Geometry check sheet. Reference: the model listing, model coordinates, mm. Give positions to 0.01 mm unless a question says otherwise; leave off trailing zeros. Order: outer loops, then holes, each group sorted by start corner. A loop starts at its lowest first (then second) coordinate and runs counter-clockwise, first axis right, second up. Notation, with made-up numbers: (-21, 79) - (20, 79) arc R28 ccw to (20, 116) - close; hole circle Ø4 at (-9.75, 61.25). An arc over 180 degrees is marked (long way). Put each result on its own line as item: value. Start each with the question number.
```python
from build123d import *

# Parameters (mm, degrees)
F0_W     = 285.75
F0_H     = 50.8
F0_R     = 2.5527
F1_DEPTH = 3.175
F3_DEPTH = 285.751


with BuildPart() as f1:
    # F0 (on Top) → F1 (new body)
    with BuildSketch(Plane.XY):
        with Locations((142.875, -25.4)):
            Rectangle(F0_W, F0_H)
        with Locations((25.4, -38.1)):
            Circle(F0_R, mode=Mode.SUBTRACT)
        with Locations((260.35, -38.1)):
            Circle(F0_R, mode=Mode.SUBTRACT)
        with Locations((25.4, -12.7)):
            Circle(F0_R, mode=Mode.SUBTRACT)
        with Locations((260.35, -12.7)):
            Circle(F0_R, mode=Mode.SUBTRACT)
    extrude(amount=F1_DEPTH)

    # F2 (on face) → F3 (cut, through all)
    with BuildSketch(Plane.YZ.offset(285.75)):
        Polygon((-50.8, 3.175), (-50.8, 0), (-34.366313, 3.175), align=None)
    extrude(amount=-F3_DEPTH, mode=Mode.SUBTRACT)


solid = f1.part
```
Item 1: Cross-section at C-C (y = -38.1). Enter the section's corners in (x, z).
Item 2: Cross-section at B-B (z = 1). Enter the section's corners in (x, y), and give its area (3 significant figures).
Item 3: Thickness scan on line 1 along X through (y, z) = (-38.1, 1.35); line 2 along X through (y, z) = (-12.5, 0.25); line 3 along Y through (x, z) = (25.4, 2.3). Record the ranges inside material, lowest first.
Item 4: Release check for a two-part mould opening along X. For faces 1 (the face through (25.07, -35.57, 1.16)), 2 (the face through (144.875, -42.698, 1.565)) record: +X half, -X half, draft (parallel to the pull), parting line (faces both ways), or undercut.
Item 5: Cross-section at A-A (x = 260.35). Enter the section's corners in (y, z) (3 decimals), and give its area (3 significant figures).
Item 6: Cross-section at D-D (x = 54.5). Enter the section's corners in (y, z) (3 decimals), and give its area (3 significant figures).
Item 7: Gauge pin test, flat end, axial feed: pin 1 Ø4.5 at (x, y) = (25.4, -38.1) entering from -Z. Record the tip position at first contact, or that the pin passes through.
Recorded:
1. outline: (0, 0) - (22.85, 0) - (22.85, 2.45) - (0, 2.45) - close; (27.95, 0) - (257.8, 0) - (257.8, 2.45) - (27.95, 2.45) - close; (262.9, 0) - (285.75, 0) - (285.75, 2.45) - (262.9, 2.45) - close
2. outline: (0, -45.62) - (285.75, -45.62) - (285.75, 0) - (0, 0) - close; hole circle Ø5.11 at (25.4, -38.1); hole circle Ø5.11 at (25.4, -12.7); hole circle Ø5.11 at (260.35, -38.1); hole circle Ø5.11 at (260.35, -12.7)
2. area: 13,000 mm^2
3. line 1: x = 0 to 22.85, 27.95 to 257.8, 262.9 to 285.75
3. line 2: x = 0 to 22.86, 27.94 to 257.81, 262.89 to 285.75
3. line 3: y = -35.55 to -15.25, -10.15 to 0
4. face 1: undercut
4. face 2: draft
5. outline: (-50.8, 0) - (-40.653, 0) - (-40.653, 1.96) - close; (-35.547, 0) - (-15.253, 0) - (-15.253, 3.175) - (-34.366, 3.175) - (-35.547, 2.947) - close; (-10.147, 0) - (0, 0) - (0, 3.175) - (-10.147, 3.175) - close
5. area: 106 mm^2
6. outline: (-50.8, 0) - (0, 0) - (0, 3.175) - (-34.366, 3.175) - close
6. area: 135 mm^2
7. pin 1: passes through
